Can you work these out from the model? Positions are in its coordinate system, mm. A direction names the side the tool comes from. Give positions to 0.01 mm unless a question says otherwise; leave off trailing zeros. Order: outer loops, then holes, each group sorted by start corner. A loop starts at its lowest first (then second) coordinate and runs counter-clockwise, first axis right, second up. Notation, with made-up numbers: M 83,29.25 L 131,29.25 A27 cw 131,58.25 Z; hole C 21,16 d10. An arc over 180 degrees is marked long. Use one line per item in the form item = value. Start each with the question number.
1. I want a section at D-D, the plane z = 4.5. List the corners of the cut face in (x, y) for me, and give its area (3 significant figures).
2. For faces 4 (the face through (-13.5, -0.5, 9.9)), 5 (the face through (-1, -1, 1)), 6 (the face through (0, 6, 0.5)), which set-ups out of +Z, -Z, +X, -X, +Y, -Y let a thin tool reach every point of the face, with its end or its side?
3. I want a section at A-A, the plane y = 3. Count the separate pieces of the cut face and the enclosed holes in it, and give its area (3 significant figures).
4. I need wall thicknesses on L1, parallel to Z at x = -11.75, y = 7.5; L2, parallel to X at y = 11.5, z = 10.5; L3, parallel to Z at x = -11.25, y = 1.25. Which ranges of each line are inside material? Lowest first, please.
5. I want a section at C-C, the plane x = -0.5. List the corners of the cut face in (y, z) for me, and give its area (3 significant figures).
6. We'd pull the mould along Z, two halves only. Please class faces 1 (the face through (15, 6, 10)), 2 (the face through (0, 6, 19.5)), 3 (the face through (0, 6, 0)): +Z half, -Z half, draft (parallel to the pull), parting line (faces both ways), or undercut.
7. Will this pin go through, and if not, where does the flat tip stop? P1, Ø2.5, axis at x = -12, y = 3, coming from the -Z side.
```python
from build123d import *

# Parameters (mm, degrees)
F0_W     = 30
F0_H     = 12
F0_R     = 1.5
F1_DEPTH = 20
F2_W     = 29
F2_H     = 19
F2_W_2   = 27
F2_H_2   = 17
F3_DEPTH = 12
F2_W_3   = 30
F2_H_3   = 20
F4_DEPTH = 1
F5_SIZE2 = 0.49999
F5_SIZE  = 0.49999


# Not quite as in the source:
# - a fillet or chamfer is up to 0.001 mm smaller than in the source, because OpenCascade refuses the exact size


with BuildPart() as f1:
    # F0 (on Top) → F1 (new body)
    with BuildSketch(Plane.XY):
        with Locations((0, 6)):
            Rectangle(F0_W, F0_H)
        with Locations((-12, 3)):
            Circle(F0_R, mode=Mode.SUBTRACT)
        with Locations((12, 3)):
            Circle(F0_R, mode=Mode.SUBTRACT)
    extrude(amount=F1_DEPTH)

    # F2 (on Front) → F3 (cut)
    with BuildSketch(Plane.XZ):
        with Locations((0, 10)):
            Rectangle(F2_W, F2_H)
        with Locations((0, 10)):
            Rectangle(F2_W_2, F2_H_2, mode=Mode.SUBTRACT)
        with Locations((0, 10)):
            Rectangle(F2_W_2, F2_H_2)
    extrude(amount=-F3_DEPTH, mode=Mode.SUBTRACT)

    # F2 (on Front) → F4 (join)
    with BuildSketch(Plane.XZ):
        with Locations((0, 10)):
            Rectangle(F2_W_3, F2_H_3)
        with Locations((0, 10)):
            Rectangle(F2_W, F2_H, mode=Mode.SUBTRACT)
        with Locations((0, 10)):
            Rectangle(F2_W, F2_H)
        with Locations((0, 10)):
            Rectangle(F2_W_2, F2_H_2, mode=Mode.SUBTRACT)
    extrude(amount=F4_DEPTH)

    # F5 (size 0.5 and 0.5 in the source; OpenCascade refuses exactly that, so slightly less here)
    f5_edges = [f1.edges().sort_by_distance(p)[0] for p in [
        (-13.5, 3, 0.5),
        (10.5, 3, 0.5),
        (10.5, 3, 19.5),
        (-13.5, 3, 19.5),
    ]]
    chamfer(f5_edges, length=F5_SIZE, length2=F5_SIZE2)


solid = f1.part
```
Check result:
q1.outline = M -15,-1 L -13.5,-1 L -13.5,0 L -14.5,0 L -14.5,12 L -15,12 Z; M 13.5,-1 L 15,-1 L 15,12 L 14.5,12 L 14.5,0 L 13.5,0 Z
q1.area = 15.0 mm2
q2.face_4 = +Y, -Y
q2.face_5 = +Z, -Z, +X, -X, -Y
q2.face_6 = +Y
q3.separate_pieces = 4
q3.enclosed_holes = 0
q3.area = 42.0 mm2
q4.L1 = 0 to 0.5, 19.5 to 20
q4.L2 = -15 to -14.5, 14.5 to 15
q4.L3 = 0 to 0.4, 19.6 to 20
q5.outline = M -1,0 L 12,0 L 12,0.5 L 0,0.5 L 0,1.5 L -1,1.5 Z; M -1,18.5 L 0,18.5 L 0,19.5 L 12,19.5 L 12,20 L -1,20 Z
q5.area = 15.0 mm2
q6.face_1 = draft
q6.face_2 = undercut
q6.face_3 = -Z half
q7.P1 = through
